```python
from build123d import *

# Parameters (mm, degrees)
EXTRUDE_1_DEPTH     = 15
SKETCH_2_R          = 2.5
CUT_EXTRUDE_1_DEPTH = 15
SKETCH_3_R          = 2.5
CUT_EXTRUDE_2_DEPTH = 15
SKETCH_4_W          = 22.93908914
SKETCH_4_H          = 7.177811465
CUT_EXTRUDE_3_DEPTH = 15
SKETCH_5_W          = 3.489667051
SKETCH_5_H          = 17.448335256
CUT_EXTRUDE_4_DEPTH = 15


with BuildPart() as part:
    # 스케치1 → 보스-돌출1 (new body)
    with BuildSketch(Plane.XY):
        Polygon((0, 0), (23, 0), (23, -23), (20, -23), (20, -3), (0, -3), align=None)
    extrude(amount=EXTRUDE_1_DEPTH)

    # 스케치2 → 컷-돌출1 (cut)
    with BuildSketch(Plane(origin=(0, 0, 0), x_dir=(1, 0, 0), z_dir=(0, 1, 0))):
        with Locations(Location((13, -7.5, 0), (0, 0, 270))):
            Circle(SKETCH_2_R)
    extrude(amount=-CUT_EXTRUDE_1_DEPTH, mode=Mode.SUBTRACT)

    # 스케치3 → 컷-돌출2 (cut)
    with BuildSketch(Plane(origin=(23, 0, 0), x_dir=(0, 0, -1), z_dir=(1, 0, 0))):
        with Locations(Location((-7.5, -10, 0), (0, 0, 90))):
            Circle(SKETCH_3_R)
    extrude(amount=-CUT_EXTRUDE_2_DEPTH, mode=Mode.SUBTRACT)

    # 스케치4 → 컷-돌출3 (cut)
    with BuildSketch(Plane(origin=(23, 0, 0), x_dir=(0, 0, -1), z_dir=(1, 0, 0))):
        with Locations((-7.664491513, -23.588905733)):
            Rectangle(SKETCH_4_W, SKETCH_4_H)
    extrude(amount=-CUT_EXTRUDE_3_DEPTH, mode=Mode.SUBTRACT)

    # 스케치5 → 컷-돌출4 (cut)
    with BuildSketch(Plane(origin=(0, 0, 0), x_dir=(1, 0, 0), z_dir=(0, 1, 0))):
        with Locations((1.255166474, -7.361337733)):
            Rectangle(SKETCH_5_W, SKETCH_5_H)
    extrude(amount=-CUT_EXTRUDE_4_DEPTH, mode=Mode.SUBTRACT)


solid = part.part
```
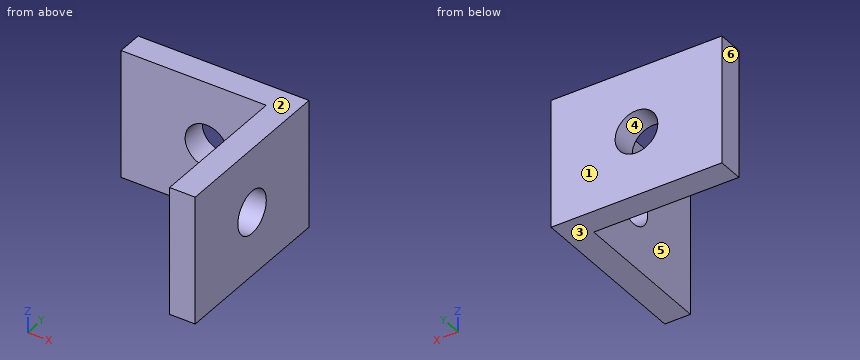
Input: part model. Units: mm. Frame: model coordinates. Face numbers are marked on the shaded views. A direction names the side the tool comes from. Coordinates: 2 decimals unless noted, no trailing zeros. Write each loop counter-clockwise with the first axis right and the second up, starting at its lowest first coordinate (ties: lowest second). Pieces come first, ordered by that corner, then holes.
1) Mould query, pull axis Z, two halves, no side actions, for the marked faces 1, 2, 3 and 4. Classes: pulls with the +Z half, pulls with the -Z half, needs draft (parallel to the pull), parting line crosses it, or undercut.
2) Material intervals for line 1 along X through (y, z) = (-1.4, 7.5); line 2 along Z through (x, y) = (22.1, -10); line 3 along Y through (x, z) = (10, 7), sorted ascending.
3) Pin query (flat end, axial travel): pin 1 Ø5 at (x, z) = (15.5, 10.5) entering from -Y; pin 2 Ø4.5 at (y, z) = (-10, 7.5) entering from -X; pin 3 Ø4.5 at (y, z) = (-11, 5) entering from -X. Return the tip coordinate at first contact, or that it passes through.
4) Set-up query: the marked faces 5 and 6. Return all of +Z, -Z, +X, -X, +Y, -Y with unobstructed straight access to the full face (end or side cutting, diameter ignored); none if empty.
5) Section C-C on z = 7.5. Output: boundary loops of the cut face in (x, y), and give its area (3 significant figures).
6) Section B-B on x = 13. Output: boundary loops of the cut face in (y, z).
7) Section D-D on x = 20.5. Output: boundary loops of the cut face in (y, z).
8) Section A-A on y = -10. Output: boundary loops of the cut face in (x, z).
Check result:
1. face 1: needs draft
1. face 2: pulls with the +Z half
1. face 3: pulls with the -Z half
1. face 4: undercut
2. line 1: x = 3 to 10.5, 15.5 to 23
2. line 2: z = 0 to 5, 10 to 15
2. line 3: y = -3 to 0
3. pin 1: stops at y = -3
3. pin 2: passes through
3. pin 3: stops at x = 20
4. face 5: +Z, -Z, -X, -Y
4. face 6: +Z, -Z, -X, +Y, -Y
5. outline: (3, -3) - (10.5, -3) - (10.5, 0) - (3, 0) - close; (15.5, -3) - (20, -3) - (20, -7.5) - (23, -7.5) - (23, 0) - (15.5, 0) - close; (20, -20) - (23, -20) - (23, -12.5) - (20, -12.5) - close
5. area: 81.0 mm2
6. outline: (-3, 0) - (0, 0) - (0, 5) - (-3, 5) - close; (-3, 10) - (0, 10) - (0, 15) - (-3, 15) - close
7. outline: (-20, 0) - (0, 0) - (0, 15) - (-20, 15) - close; hole circle Ø5 at (-10, 7.5)
8. outline: (20, 0) - (23, 0) - (23, 5) - (20, 5) - close; (20, 10) - (23, 10) - (23, 15) - (20, 15) - close
